Verification items for the finished model (mm, model axes). A direction names the side the tool comes from. Round coordinates to 2 decimals unless told otherwise and drop trailing zeros. Write each loop counter-clockwise with the first axis right and the second up, starting at its lowest first coordinate (ties: lowest second). Pieces come first, ordered by that corner, then holes. Notation, with made-up numbers: (36.5, 49.5) - (63.5, 49.5) arc R6 ccw to (63.5, 60.5) - close; hole circle Ø9 at (8.25, 7). An arc over 180 degrees is marked (long way). Write each question's results on one line, items separated by ' | '.
```python
from build123d import *

# Parameters (mm, degrees)
SKETCH1_R           = 10
BOSS_EXTRUDE1_DEPTH = 4.75
SKETCH3_R           = 1.75
CUT_EXTRUDE1_DEPTH  = 4.75


with BuildPart() as part:
    # Sketch1 → Boss-Extrude1 (new body)
    with BuildSketch(Plane(origin=(0, 0, 0), x_dir=(1, 0, 0), z_dir=(0, 1, 0))):
        with Locations(Location((0, 0, 0), (0, 0, 270))):
            Circle(SKETCH1_R)
    extrude(amount=BOSS_EXTRUDE1_DEPTH)

    # Sketch2 → Cut-Revolve1 (revolve, cut)
    with BuildSketch(Plane(origin=(0, 0, 0), x_dir=(0, 0, -1), z_dir=(1, 0, 0)), mode=Mode.PRIVATE) as cut_revolve1_sk:
        Polygon((9.578947368, 4.25), (8, 2.375), (9.578947368, 0.5), (10, 0.5), (10, 4.25), align=None)
    revolve(cut_revolve1_sk.sketch.rotate(Axis((0, 4.75, 0), (0, -1, 0)), 180), axis=Axis((0, 4.75, 0), (0, -1, 0)), mode=Mode.SUBTRACT)

    # Sketch3 → Cut-Extrude1 (cut)
    with BuildSketch(Plane(origin=(0, 4.75, 0), x_dir=(1, 0, 0), z_dir=(0, 1, 0))):
        with Locations(Location((0, 0, 0), (0, 0, 270))):
            Circle(SKETCH3_R)
    extrude(amount=-CUT_EXTRUDE1_DEPTH, mode=Mode.SUBTRACT)


solid = part.part
```
(1) Section check C-C (y = 3.5). Record the cut outline in (x, z), plus the area to 3 significant figures.
Answer:
outline: circle Ø17.89 at (0, 0); hole circle Ø3.5 at (0, 0) | area: 242 mm2
(2) Section check B-B (z = 0). Record the cut outline in (x, y) (3 decimals), plus the area to 3 significant figures.
Answer:
outline: (-10, 0) - (-1.75, 0) - (-1.75, 4.75) - (-10, 4.75) - (-10, 4.25) - (-9.579, 4.25) - (-8, 2.375) - (-9.579, 0.5) - (-10, 0.5) - close; (1.75, 0) - (10, 0) - (10, 0.5) - (9.579, 0.5) - (8, 2.375) - (9.579, 4.25) - (10, 4.25) - (10, 4.75) - (1.75, 4.75) - close | area: 69.3 mm2
(3) Set-up check for faces 4 (the flat face through (0, 0, 2)), 5 (the conical face through (7.906, 2.258, -1.756)): record each of +Z, -Z, +X, -X, +Y, -Y from which the full face is reachable in a straight line by a thin tool's end or side.
Answer:
face 4: +Z, -Z, +X, -X, -Y | face 5: none
(4) Section check A-A (x = 0). Record the cut outline in (y, z) (3 decimals).
Answer:
outline: (0, -10) - (0.5, -10) - (0.5, -9.579) - (2.375, -8) - (4.25, -9.579) - (4.25, -10) - (4.75, -10) - (4.75, -1.75) - (0, -1.75) - close; (0, 1.75) - (4.75, 1.75) - (4.75, 10) - (4.25, 10) - (4.25, 9.579) - (2.375, 8) - (0.5, 9.579) - (0.5, 10) - (0, 10) - close
(5) Mould release check, pull along Z, two halves, no side actions. Record for faces 1 (the cylindrical face through (-1.71, 2.41, -0.38)), 2 (the cylindrical face through (-9.76, 4.5, -2.17)), 3 (the flat face through (0, 4.75, 2)): released by +Z, released by -Z, zero draft, split by the parting line, or undercut.
Answer:
face 1: undercut | face 2: split by the parting line | face 3: zero draft
(6) Go/stop test with flat-tipped pins: pin 1 Ø2 at (y, z) = (4, 5.5) entering from +X; pin 2 Ø1 at (y, z) = (1.5, 4.5) entering from -X; pin 3 Ø1 at (x, y) = (6.5, 3.5) entering from +Z. Record where each tip stops, or that it passes through.
Answer:
pin 1: x = 8.91 | pin 2: x = -8.05 | pin 3: z = 6.91
(7) Thickness scan on L1, parallel to Y at x = -8.5, z = 4.75; L2, parallel to Y at x = -2.75, z = 8.5; L3, parallel to X at y = 3.8, z = 0. Record the ranges inside material, lowest first.
Answer:
L1: 0 to 0.5, 4.25 to 4.75 | L2: 0 to 1.27, 3.48 to 4.75 | L3: -9.2 to -1.75, 1.75 to 9.2
